```python
from build123d import *

# Parameters (mm, degrees)
SKETCH_1_W          = 150
SKETCH_1_H          = 200
EXTRUDE_1_DEPTH     = 4
SKETCH_2_R          = 1.6
SKETCH_2_R_2        = 2.75
SKETCH_2_R_3        = 2.1
SKETCH_2_W          = 3.58217065
SKETCH_2_H          = 37.507433864
CUT_EXTRUDE_1_DEPTH = 5


with BuildPart() as part:
    # 草图1 → 凸台-拉伸1 (new body)
    with BuildSketch(Plane(origin=(0, 0, 0), x_dir=(1, 0, 0), z_dir=(0, 1, 0))):
        with Locations((0, -30)):
            Rectangle(SKETCH_1_W, SKETCH_1_H)
    extrude(amount=EXTRUDE_1_DEPTH)

    # 草图2 → 切除-拉伸1 (cut, through all)
    with BuildSketch(Plane(origin=(0, 4, 0), x_dir=(1, 0, 0), z_dir=(0, 1, 0))):
        with Locations((-66.052318668, 65)):
            Circle(SKETCH_2_R)
        with Locations((-66.052318668, 35)):
            Circle(SKETCH_2_R)
        with Locations((-42.052318668, 65)):
            Circle(SKETCH_2_R)
        with Locations((-42.052318668, 35)):
            Circle(SKETCH_2_R)
        with Locations((42.052318668, 35)):
            Circle(SKETCH_2_R)
        with Locations((66.052318668, 35)):
            Circle(SKETCH_2_R)
        with Locations((66.052318668, 65)):
            Circle(SKETCH_2_R)
        with Locations((42.052318668, 65)):
            Circle(SKETCH_2_R)
        with Locations((-23, -90)):
            Circle(SKETCH_2_R_2)
        with Locations((-23, -116)):
            Circle(SKETCH_2_R_2)
        with Locations((-69, -101)):
            Circle(SKETCH_2_R_3)
        with Locations((-69, -125)):
            Circle(SKETCH_2_R_3)
        with Locations((69, -125)):
            Circle(SKETCH_2_R_3)
        with Locations((69, -101)):
            Circle(SKETCH_2_R_3)
        with Locations((23, -116)):
            Circle(SKETCH_2_R_2)
        with Locations((23, -90)):
            Circle(SKETCH_2_R_2)
        with Locations((-39, -125)):
            Circle(SKETCH_2_R_3)
        with Locations((-39, -101)):
            Circle(SKETCH_2_R_3)
        with Locations((39, -125)):
            Circle(SKETCH_2_R_3)
        with Locations((39, -101)):
            Circle(SKETCH_2_R_3)
        with Locations((-60, 5)):
            Circle(SKETCH_2_R)
        with Locations((-60, -53)):
            Circle(SKETCH_2_R)
        with Locations((-11, -53)):
            Circle(SKETCH_2_R)
        with Locations((-11, 5)):
            Circle(SKETCH_2_R)
        with Locations((20, 5)):
            Circle(SKETCH_2_R)
        with Locations((60, 5)):
            Circle(SKETCH_2_R)
        with Locations((20, -40)):
            Circle(SKETCH_2_R)
        with Locations((60, -40)):
            Circle(SKETCH_2_R)
        with BuildLine():
            Line((-1.6, -123.5), (-1.6, -125.5))
            ThreePointArc((-1.6, -125.5), (0, -127.1), (1.6, -125.5))
            Line((1.6, -125.5), (1.6, -123.5))
            ThreePointArc((1.6, -123.5), (0, -121.9), (-1.6, -123.5))
        make_face()
        with BuildLine():
            Line((-1.6, -113.5), (-1.6, -115.5))
            ThreePointArc((-1.6, -115.5), (0, -117.1), (1.6, -115.5))
            Line((1.6, -115.5), (1.6, -113.5))
            ThreePointArc((1.6, -113.5), (0, -111.9), (-1.6, -113.5))
        make_face()
        with Locations((-22.068717893, 42.893406935)):
            Rectangle(SKETCH_2_W, SKETCH_2_H)
    extrude(amount=-CUT_EXTRUDE_1_DEPTH, mode=Mode.SUBTRACT)


solid = part.part
```
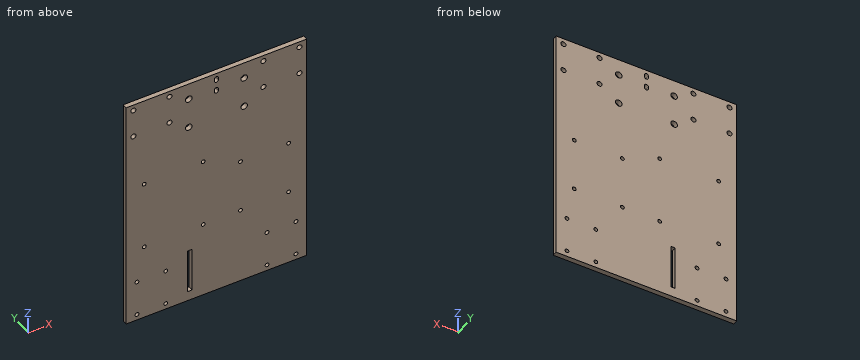
The listing builds one solid part. Answer for the finished solid, in the listing's coordinates (mm). Coordinates: 2 decimals unless noted, no trailing zeros. Write each loop counter-clockwise with the first axis right and the second up, starting at its lowest first coordinate (ties: lowest second). Pieces come first, ordered by that corner, then holes. Notation, with made-up numbers: (-36.75, 17.25) - (7.25, 17.25) arc R27 ccw to (7.25, 55.25) - close; hole circle Ø5 at (16.5, 7.5). An arc over 180 degrees is marked (long way). Return JSON: item names as keys, results as strings. Group by question number.
Q1. The part is cut by section A-A on z = -53.5. Write down the section's boundary in (x, y).
Q2. The part is cut by section B-B on y = 3.2. State how many separate pieces and enclosed holes the cut face has, and give its area (3 significant figures).
Q3. Find the intervals of material crossed by line 1 along X through (y, z) = (1.75, -5); line 2 along X through (y, z) = (3.2, 125); line 3 along Z through (x, y) = (23, 1.1), in increasing order. Write a range as [from, to].
Evaluation:
{
 "1": {"outline": "(-75, 0) - (-23.86, 0) - (-23.86, 4) - (-75, 4) - close; (-20.28, 0) - (75, 0) - (75, 4) - (-20.28, 4) - close"},
 "2": {"separate pieces": "1", "enclosed holes": "31", "area": "29,500 mm2"},
 "3": {"line 1": "x = [-75, -61.6], [-58.4, -12.6], [-9.4, 18.4], [21.6, 58.4], [61.6, 75]", "line 2": "x = [-75, -71.1], [-66.9, -41.1], [-36.9, -1.6], [1.6, 36.9], [41.1, 66.9], [71.1, 75]", "line 3": "z = [-70, 87.25], [92.75, 113.25], [118.75, 130]"}
}
